from build123d import *

# Parameters (mm, degrees)
CROQUIS1_W              = 60
CROQUIS1_H              = 25
SALIENTE_EXTRUIR1_DEPTH = 5
CROQUIS2_W              = 20
CROQUIS2_H              = 3
SALIENTE_EXTRUIR2_DEPTH = 10
CROQUIS3_W              = 60
CROQUIS3_H              = 25
CORTAR_EXTRUIR1_DEPTH   = 2
CROQUIS4_W              = 20
CROQUIS4_H              = 3
SALIENTE_EXTRUIR3_DEPTH = 5


with BuildPart() as part:
    # Croquis1 → Saliente-Extruir1 (new body)
    with BuildSketch(Plane.XY):
        Rectangle(CROQUIS1_W, CROQUIS1_H)
    extrude(amount=SALIENTE_EXTRUIR1_DEPTH)

    # Croquis2 → Saliente-Extruir2 (add)
    with BuildSketch(Plane(origin=(0, 0, 0), x_dir=(-1, 0, 0), z_dir=(0, 0, -1))):
        Rectangle(CROQUIS2_W, CROQUIS2_H)
    extrude(amount=SALIENTE_EXTRUIR2_DEPTH)

    # Croquis3 → Cortar-Extruir1 (cut)
    with BuildSketch(Plane.XY.offset(5)):
        Rectangle(CROQUIS3_W, CROQUIS3_H)
    extrude(amount=-CORTAR_EXTRUIR1_DEPTH, mode=Mode.SUBTRACT)

    # Croquis4 → Saliente-Extruir3 (add)
    with BuildSketch(Plane(origin=(0, 0, -10), x_dir=(-1, 0, 0), z_dir=(0, 0, -1))):
        Rectangle(CROQUIS4_W, CROQUIS4_H)
    extrude(amount=SALIENTE_EXTRUIR3_DEPTH)


solid = part.part
The model under review builds one solid part; all positions refer to its coordinate system, in mm. A direction names the side the tool comes from. Round coordinates to 2 decimals unless told otherwise and drop trailing zeros. Order: outer loops, then holes, each group sorted by start corner. A loop starts at its lowest first (then second) coordinate and runs counter-clockwise, first axis right, second up. Notation, with made-up numbers: (5, -40) - (25, -40) arc R23 cw to (25, -28) - close; hole circle Ø5 at (-33.5, 14). An arc over 180 degrees is marked (long way). Use one line per item in the form item = value.
Q1. Clearance check with flat-ended pins moving along their axes: P1, Ø1, axis at x = -9, z = -13, coming from the +Y side; P2, Ø2.5, axis at y = 0.5, z = -7, coming from the +X side; P3, Ø1.5, axis at y = 0.5, z = -1.5, coming from the -X side. State where each tip first meets the part, or that it passes through.
Response values:
P1 = 1.5
P2 = 10
P3 = -10
Q2. Add section D-D on y = 5.5. Give the boundary of the cut face in (x, z).
Response values:
outline = (-30, 0) - (30, 0) - (30, 3) - (-30, 3) - close
Q3. Add section A-A on y = 0. Give the boundary of the cut face in (x, z), then the cut area to 3 significant figures.
Response values:
outline = (-30, 0) - (-10, 0) - (-10, -15) - (10, -15) - (10, 0) - (30, 0) - (30, 3) - (-30, 3) - close
area = 480 mm^2
Q4. Add section C-C on z = -9.75. Give the boundary of the cut face in (x, y), then the cut area to 3 significant figures.
Response values:
outline = (-10, -1.5) - (10, -1.5) - (10, 1.5) - (-10, 1.5) - close
area = 60.0 mm^2
Q5. To check wall thickness, follow line 1 (Z direction, x = 14, y = -2); line 2 (X direction, y = 0.75, z = -0.75); line 3 (Y direction, x = -4, z = -8.5). State the ranges of each line that lie inside material, in increasing order.
Response values:
line_1 = 0 to 3
line_2 = -10 to 10
line_3 = -1.5 to 1.5
Q6. Tool access review of faces 1 (the flat face through (0, 1.5, -7)), 2 (the flat face through (10, 0, -7)), 3 (the flat face through (-10, 0, -7)), 4 (the flat face through (0, -1.5, -7)): name each direction out of +Z, -Z, +X, -X, +Y, -Y from which nothing blocks a thin tool from reaching the whole face with its end or side.
Response values:
face_1 = -Z, +X, -X, +Y
face_2 = -Z, +X, +Y, -Y
face_3 = -Z, -X, +Y, -Y
face_4 = -Z, +X, -X, -Y
Q7. Add section B-B on x = 6. Give the boundary of the cut face in (y, z), then the cut area to 3 significant figures.
Response values:
outline = (-12.5, 0) - (-1.5, 0) - (-1.5, -15) - (1.5, -15) - (1.5, 0) - (12.5, 0) - (12.5, 3) - (-12.5, 3) - close
area = 120 mm^2
